Study the drawing (mm; zero at the part's minimum x, y, z) and answer. Coordinates: 2 decimals unless noted, no trailing zeros. Loops run counter-clockwise (first coordinate to the right, second up) from the corner with the lowest first, then second, coordinate; pieces in that order, holes last. Notation, with made-up numbers: (50.25, 17.5) -> (92.25, 17.5) arc R14 ccw to (92.25, 38.5) -> close; hole circle Ø10 at (-14.75, -36). An arc over 180 degrees is marked (long way). Answer as a JSON object with one key per item and string values. Group by question number.
Q1. The part is cut by section B-B on z = 22.5. Write down the section's boundary in (x, y), and give its area (3 significant figures).
Q2. The part is cut by section A-A on x = 1.7. Write down the section's boundary in (y, z), and give its area (3 significant figures).
Q3. Straight lines are drawn through the part: line 1 along Z through (x, y) = (0.5, 17); line 2 along Y through (x, z) = (2.15, 19.5). For each, find the intervals that lie inside material, in ascending order. Write a range as [from, to].
Q4. The part is cut by section C-C on y = 52. Write down the section's boundary in (x, z).
Q5. Each of these flat-tipped pins is pushed along its axis until it touches: P1, Ø0.8, axis at x = 1, z = 100, coming from the +Y side; P2, Ø1.3, axis at x = 1, y = 1, coming from the +Z side; P3, Ø0.8, axis at x = 1, z = 101, coming from the -Y side. Where does it stop, or does it pass through?
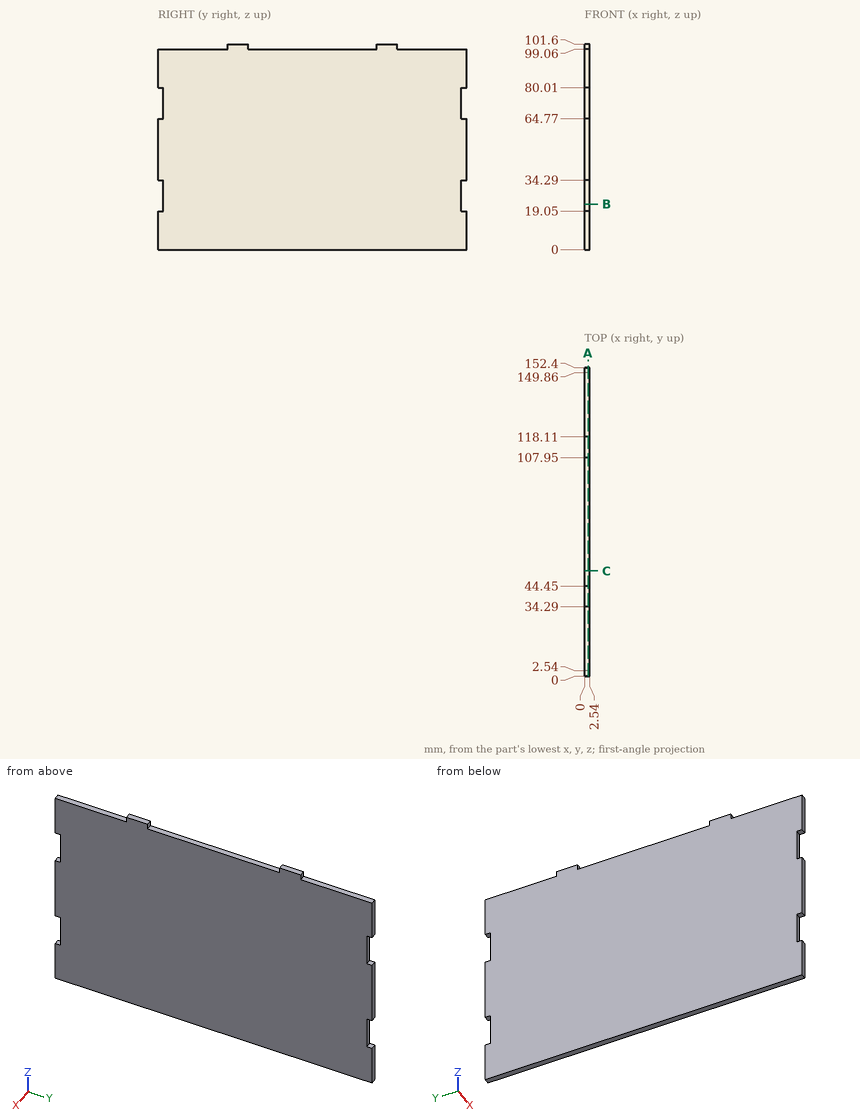
Final values:
{
 "1": {"outline": "(0, 2.54) -> (2.54, 2.54) -> (2.54, 149.86) -> (0, 149.86) -> close", "area": "374 mm2"},
 "2": {"outline": "(0, 0) -> (152.4, 0) -> (152.4, 19.05) -> (149.86, 19.05) -> (149.86, 34.29) -> (152.4, 34.29) -> (152.4, 64.77) -> (149.86, 64.77) -> (149.86, 80.01) -> (152.4, 80.01) -> (152.4, 99.06) -> (118.11, 99.06) -> (118.11, 101.6) -> (107.95, 101.6) -> (107.95, 99.06) -> (44.45, 99.06) -> (44.45, 101.6) -> (34.29, 101.6) -> (34.29, 99.06) -> (0, 99.06) -> (0, 80.01) -> (2.54, 80.01) -> (2.54, 64.77) -> (0, 64.77) -> (0, 34.29) -> (2.54, 34.29) -> (2.54, 19.05) -> (0, 19.05) -> close", "area": "15,000 mm2"},
 "3": {"line 1": "z = [0, 99.06]", "line 2": "y = [2.54, 149.86]"},
 "4": {"outline": "(0, 0) -> (2.54, 0) -> (2.54, 99.06) -> (0, 99.06) -> close"},
 "5": {"P1": "stops at y = 118.11", "P2": "stops at z = 99.06", "P3": "stops at y = 34.29"}
}
